Drawing for the job (mm, zero at the part's lowest x, y, z). Round coordinates to 2 decimals unless told otherwise and drop trailing zeros. Order: outer loops, then holes, each group sorted by start corner. A loop starts at its lowest first (then second) coordinate and runs counter-clockwise, first axis right, second up. Notation, with made-up numbers: M 66.5,29.5 L 82.5,29.5 A22 ccw 82.5,54.5 Z; hole C 5,10.5 d3. An arc over 180 degrees is marked long. One line per item, written item: value. Start each with the question number.
Item 1: Band-saw the part on C-C, the plane y = 21. Write the cut outline in (x, z) (3 decimals), then the cut area to 3 significant figures.
Item 2: Band-saw the part on B-B, the plane z = 6.75. Write the cut outline in (x, y), then the cut area to 3 significant figures.
Item 3: Pin check, flat tips, straight feed: pin 1 (11.5 mm diameter, centred on x = 28, y = 21, fed in from +Z); pin 2 (3 mm diameter, centred on y = 23.5, z = 8.5, fed in from +X); pin 3 (2 mm diameter, centred on y = 31.5, z = 6, fed in from +X). Stop position of each tip, or through.
Item 4: Band-saw the part on D-D, the plane x = 70. Write the cut outline in (y, z).
Item 5: Band-saw the part on A-A, the plane x = 28. Write the cut outline in (y, z) (3 decimals), then the cut area to 3 significant figures.
Item 6: Two-plate mould, pull along Y, no slides. Class the marked faces 1, 2, 3 and 4: +Y half, -Y half, draft (parallel to the pull), parting line (faces both ways), or undercut.
Item 7: Probe L1, parallel to Y at x = 28, z = 13.1 (3 decimals); L2, parallel to Y at x = 28, z = 5.5; L3, parallel to Y at x = 37.5, z = 13.25. List the from-to ranges inside material, lowest first.
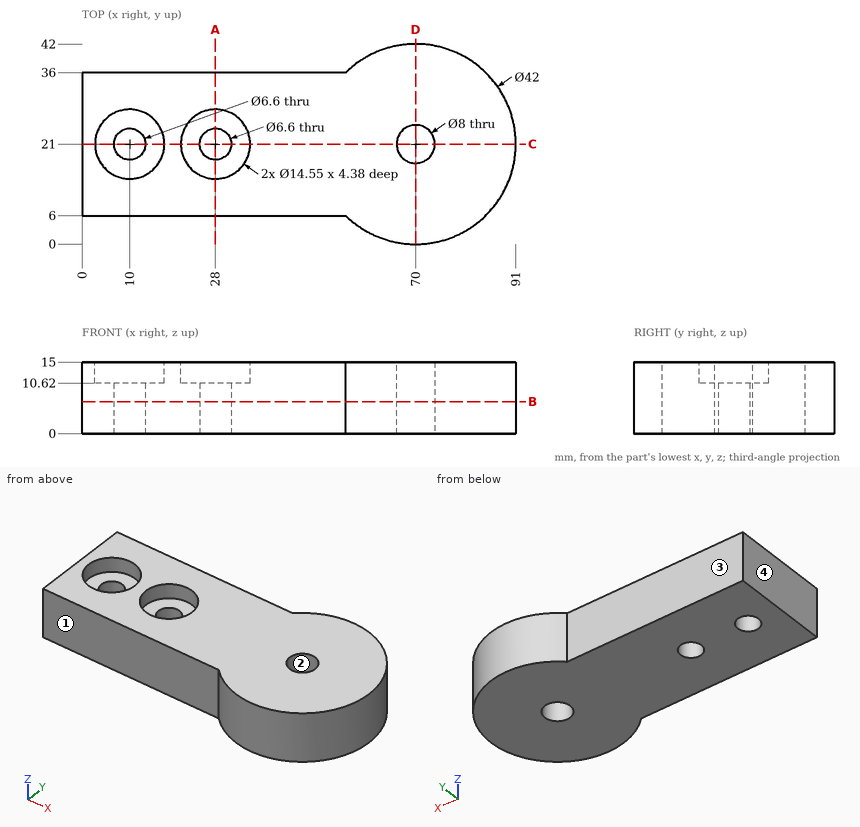
Output:
1. outline: M 0,0 L 6.7,0 L 6.7,10.62 L 2.725,10.62 L 2.725,15 L 0,15 Z; M 13.3,0 L 24.7,0 L 24.7,10.62 L 20.725,10.62 L 20.725,15 L 17.275,15 L 17.275,10.62 L 13.3,10.62 Z; M 31.3,0 L 66,0 L 66,15 L 35.275,15 L 35.275,10.62 L 31.3,10.62 Z; M 74,0 L 91,0 L 91,15 L 74,15 Z
1. area: 977 mm²
2. outline: M 0,6 L 55.3,6 A21 ccw long 55.3,36 L 0,36 Z; hole C 10,21 d6.6; hole C 28,21 d6.6; hole C 70,21 d8
2. area: 2,800 mm²
3. pin 1: stops at z = 10.62
3. pin 2: stops at x = 90.98
3. pin 3: stops at x = 88.73
4. outline: M 0,0 L 17,0 L 17,15 L 0,15 Z; M 25,0 L 42,0 L 42,15 L 25,15 Z
5. outline: M 6,0 L 17.7,0 L 17.7,10.62 L 13.725,10.62 L 13.725,15 L 6,15 Z; M 24.3,0 L 36,0 L 36,15 L 28.275,15 L 28.275,10.62 L 24.3,10.62 Z
5. area: 316 mm²
6. face 1: -Y half
6. face 2: undercut
6. face 3: +Y half
6. face 4: draft
7. L1: y = 6 to 13.725, 28.275 to 36
7. L2: y = 6 to 17.7, 24.3 to 36
7. L3: y = 6 to 36
